Can you work these out from the model? Positions are in its coordinate system, mm. A direction names the side the tool comes from. Coordinates: 2 decimals unless noted, no trailing zeros.
```python
from build123d import *

# Parameters (mm, degrees)
ESQUISSE2_R           = 1.25
EXTRUSION1_DEPTH      = 10
BALAYAGE1_PITCH       = 2.5
EXTRUSION2_DEPTH      = 20.313652943
EXTRUSION2_DEPTH_BACK = 3
ESQUISSE5_R           = 3.615449726


with BuildPart() as part:
    # Esquisse2 → Extrusion1 (new body)
    with BuildSketch(Plane.XZ.offset(-4.657558322)):
        with Locations(Location((-0.389434894, -13.47998185, 0), (0, 0, 270))):
            Circle(ESQUISSE2_R)
    extrude(amount=EXTRUSION1_DEPTH)

    # Balayage1: the profile of Esquisse4 profile screwed along a right-hand helix of 4 turns, 10 arcs to a turn; built about Z, then put on its axis
    balayage1_z = Axis((0, 0, 0), (0, 0, 1))
    balayage1_corners = [(2.5, 0, 0), (1.2497, 0, 0.455071984), (1.2497, 0, -0.455071984)]
    with BuildLine(mode=Mode.PRIVATE) as balayage1_profile:
        Line(balayage1_corners[0], balayage1_corners[1])
        Line(balayage1_corners[1], balayage1_corners[2])
        Line(balayage1_corners[2], balayage1_corners[0])
    balayage1_cap = Face(balayage1_profile.wire())
    balayage1_turn_angles = [0, 18, 36, 54, 72, 90, 108, 126, 144, 162, 180, 198, 216, 234, 252, 270, 288, 306, 324, 342, 360]
    balayage1_turn_weights = [1, 0.9510565162951535, 1, 0.9510565162951535, 1, 0.9510565162951535, 1, 0.9510565162951535, 1, 0.9510565162951535, 1, 0.9510565162951535, 1, 0.9510565162951535, 1, 0.9510565162951535, 1, 0.9510565162951535, 1, 0.9510565162951535, 1]
    balayage1_turn_rails = [Edge.make_bspline([Vector(p[0], p[1], 0).rotate(balayage1_z, balayage1_turn_angles[k]) / balayage1_turn_weights[k] + Vector(0, 0, p[2] + BALAYAGE1_PITCH * balayage1_turn_angles[k] / 360) for k in range(21)], [0, 0, 0, 1, 1, 2, 2, 3, 3, 4, 4, 5, 5, 6, 6, 7, 7, 8, 8, 9, 9, 10, 10, 10], 2, balayage1_turn_weights) for p in balayage1_corners]
    balayage1_turn_sides = [Face.make_surface_from_curves(balayage1_turn_rails[p[0]], balayage1_turn_rails[p[1]]) for p in [(0, 1), (1, 2), (2, 0)]]
    balayage1 = Plane(origin=(-0.389434894, -5.342441678, -13.47998185), x_dir=(0, 0, -1), z_dir=(0, 1, 0)) * Solid(Shell([*[p.moved(Location((0, 0, BALAYAGE1_PITCH * i))) for i in range(4) for p in balayage1_turn_sides], balayage1_cap, balayage1_cap.rotate(balayage1_z, 1440).moved(Location((0, 0, BALAYAGE1_PITCH * 1440 / 360)))]))
    add(balayage1)

    # Esquisse5 → Extrusion2 (cut, two sides: drawn at the far end of the back side and taken through both)
    with BuildSketch(Plane.XZ.offset(5.342441678).offset(-EXTRUSION2_DEPTH_BACK)):
        with Locations((-0.389434894, -13.47998185)):
            Circle(ESQUISSE5_R)
    extrude(amount=EXTRUSION2_DEPTH + EXTRUSION2_DEPTH_BACK, mode=Mode.SUBTRACT)


solid = part.part
```
1. I'm going to push flat-ended pins straight in: pin 1 (0.8 mm diameter, centred on x = -1, z = -14, fed in from +Y); pin 2 (1 mm diameter, centred on x = -0.5, y = -1.5, fed in from -Z); pin 3 (1 mm diameter, centred on x = -1.5, y = 3.5, fed in from -Z). Where does each tip first touch, or does it pass through?
Completed:
pin 1: stops at y = 4.66
pin 2: stops at z = -14.73
pin 3: stops at z = -14.57
2. Please list where these lines run through material, in increasing order: probe 1 along Y at (x, z) = (-0.1, -15.7); probe 2 along Y at (x, z) = (-1.55, -14.5); probe 3 along X at (y, z) = (3.25, -13.55).
Completed:
probe 1: y = -0.49 to -0.3, 2.01 to 2.2, 4.51 to 4.7
probe 2: y = -2.34 to -2.16, -0.35 to 0.34, 2.15 to 2.84
probe 3: x = -1.64 to 0.86
3. Imagine slicing it at A-A on z = -15.55. Give the number of separate pieces and of enclosed holes in the cut face, then the cut area to 3 significant figures.
Completed:
separate pieces: 3
enclosed holes: 0
area: 1.43 mm2
4. On a 3-axis mill with a long thin cutter (end or side, diameter ignored), from which of +Z, -Z, +X, -X, +Y, -Y can I reach the whole of each face in a straight line? I mean faces 1 (the flat face through (-0.389, 4.7, -15.2)), 2 (the flat face through (-1, -2.342, -14)), 3 (the flat face through (0, 4.658, -13)). Say none if no direction works.
Completed:
face 1: -Z, -X, +Y
face 2: +Z, -Z, +X, -X, -Y
face 3: +Z, -X, +Y
